Build history of the part. All positions in model axes, mm. Face numbers are marked on the shaded views. A direction names the side the tool comes from. Give positions to 0.01 mm unless a question says otherwise; leave off trailing zeros. Order: outer loops, then holes, each group sorted by start corner. A loop starts at its lowest first (then second) coordinate and runs counter-clockwise, first axis right, second up. Notation, with made-up numbers: (-19.75, 20.5) - (18.25, 20.5) arc R28 cw to (18.25, 47.5) - close; hole circle Ø4 at (-6.5, -13). An arc over 180 degrees is marked (long way). Use a Markdown table: item, result. Add a question column.
(1) Flat gauge pins, fed straight in: pin 1 (5 mm diameter, centred on y = -36, z = 26, fed in from -X); pin 2 (12.5 mm diameter, centred on x = -93, z = 32, fed in from -Y); pin 3 (8 mm diameter, centred on y = -31.5, z = 24, fed in from +X). Where does each tip first touch, or does it go through?
(2) Slice it at A-A (x = -13). Write the cut outline in (y, z).
(3) Slice it at C-C (z = 70.5). Write the cut outline in (x, y).
(4) Wall check: line 1 (Z direction, x = -10, y = -51.5); line 2 (Y direction, x = -14, z = 5); line 3 (Z direction, x = -89, y = -79). Give the ranges that are in metal, low to high.
(5) Mould opens along Z. For the marked faces 1, 2, 3 and 4 say: +Z half, -Z half, draft (parallel to the pull), parting line (faces both ways), or undercut.
(6) Which spindle directions (+Z, -Z, +X, -X, +Y, -Y) get a long thin tool onto all of the face, cutting with end or side? Do the marked faces 5, 6 and 7. Say none if no direction does.
(7) Slice it at B-B (y = -50). Write the cut outline in (x, z), then the cut area to 3 significant figures.
from build123d import *

# Parameters (mm, degrees)
F0_W     = 101.6
F0_H     = 101.6
F1_DEPTH = 101.6
F2_W     = 25.4
F2_H     = 101.6
F3_DEPTH = 74.422
F4_W     = 101.205684
F4_H     = 74.202821
F5_DEPTH = 7.874
F7_DEPTH = 102.616
F9_DEPTH = 25.4


with BuildPart() as f1:
    # F0 (on Top) → F1 (new body)
    with BuildSketch(Plane.XY):
        with Locations((-50.8, -50.8)):
            Rectangle(F0_W, F0_H)
    extrude(amount=F1_DEPTH)

    # F2 (on face) → F3 (cut)
    with BuildSketch(Plane.XZ.offset(101.6)):
        with Locations((-12.7, 50.8)):
            Rectangle(F2_W, F2_H)
        with Locations((-88.9, 50.8)):
            Rectangle(F2_W, F2_H)
    extrude(amount=-F3_DEPTH, mode=Mode.SUBTRACT)

    # F4 (on Top) → F5 (join)
    with BuildSketch(Plane.XY):
        with Locations((-50.602842, -64.534433)):
            Rectangle(F4_W, F4_H)
    extrude(amount=F5_DEPTH)

    # F6 (on face) → F7 (cut)
    with BuildSketch(Plane.YZ.offset(-25.4)):
        Polygon((-101.6, 101.6), (-101.6, 7.874), (-27.178, 77.03993), (-27.178, 101.6), align=None)
    extrude(amount=-F7_DEPTH, mode=Mode.SUBTRACT)

    # F8 (on face) → F9 (join)
    with BuildSketch(Plane.XZ.offset(27.178)):
        Polygon((0, 101.6), (-101.6, 101.6), (-101.6, 77.03993), (-76.2, 77.03993), (-25.4, 77.03993), (0, 77.03993), align=None)
    extrude(amount=F9_DEPTH)


solid = f1.part
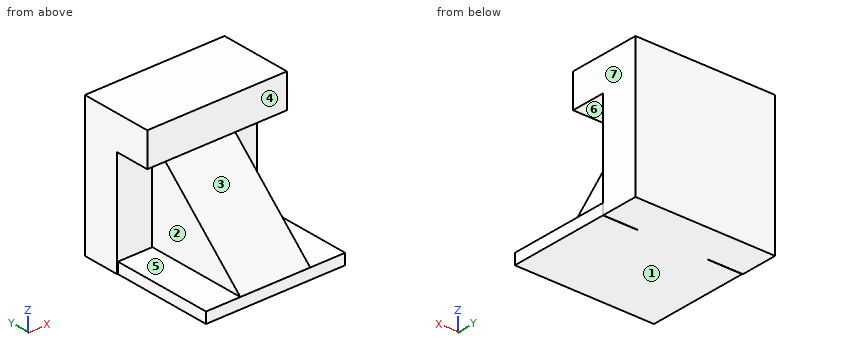
Solution:
| question | item | result |
|---|---|---|
| 1 | pin 1 | x = -76.2 |
| 1 | pin 2 | y = -27.18 |
| 1 | pin 3 | x = -25.4 |
| 2 | outline | (-101.64, 0) - (-27.43, 0) - (-27.43, 7.87) - (-101.64, 7.87) - close; (-52.58, 77.04) - (-27.18, 77.04) - (-27.18, 0) - (0, 0) - (0, 101.6) - (-52.58, 101.6) - close |
| 3 | outline | (-101.6, -27.18) - (-76.2, -27.18) - (-76.2, -34.21) - (-25.4, -34.21) - (-25.4, -27.18) - (0, -27.18) - (0, 0) - (-101.6, 0) - close |
| 4 | line 1 | 0 to 7.87, 77.04 to 101.6 |
| 4 | line 2 | -101.64 to -27.43, -27.18 to 0 |
| 4 | line 3 | 0 to 7.87 |
| 5 | face 1 | -Z half |
| 5 | face 2 | undercut |
| 5 | face 3 | undercut |
| 5 | face 4 | draft |
| 6 | face 5 | -Y |
| 6 | face 6 | +X, -X, -Y |
| 6 | face 7 | +Z, -Z, +X, +Y, -Y |
| 7 | outline | (-101.6, 77.04) - (0, 77.04) - (0, 101.6) - (-101.6, 101.6) - close; (-101.21, 0) - (0, 0) - (0, 7.87) - (-25.4, 7.87) - (-25.4, 55.83) - (-76.2, 55.83) - (-76.2, 7.87) - (-101.21, 7.87) - close |
| 7 | area | 5,730 mm2 |
